```python
from build123d import *

# Parameters (mm, degrees)
F0_W      = 38.1
F0_H      = 6.35
F1_DEPTH  = 546.1
F3_DEPTH  = 12.7
F4_W      = 152.376732
F4_H      = 158.75
F5_DEPTH  = 50.8
F6_W      = 158.75
F6_H      = 12.7
F7_DEPTH  = 152.4
F8_W      = 6.35
F8_H      = 158.75
F9_DEPTH  = 12.7
F11_DEPTH = 152.4
F12_W     = 292.1
F12_H     = 44.45
F13_DEPTH = 139.7
F14_W     = 292.1
F14_H     = 44.45
F14_W_2   = 25.4
F14_H_2   = 12.7
F15_DEPTH = 6.35


with BuildPart() as f1:
    # F0 (on Top) → F1 (new body)
    with BuildSketch(Plane.XY):
        Polygon((-59.489019, 112.964728), (-59.489019, 100.264728), (-21.389019, 100.264728), (54.810981, 100.264728), (92.910981, 100.264728), (92.910981, 112.964728), align=None)
        with Locations((73.860981, 97.089728)):
            Rectangle(F0_W, F0_H)
        Polygon((92.910981, 93.914728), (54.810981, 93.914728), (42.110981, 93.914728), (42.110981, 68.514728), (92.910981, 68.514728), align=None)
        with Locations((-40.439019, 97.089728)):
            Rectangle(F0_W, F0_H)
        Polygon((-59.489019, 93.914728), (-59.489019, 68.514728), (-8.689019, 68.514728), (-8.689019, 93.914728), (-21.389019, 93.914728), align=None)
    extrude(amount=F1_DEPTH)

    # F2 (on face) → F3 (join)
    with BuildSketch(Plane(origin=(0, 0, 0), x_dir=(1, 0, 0), z_dir=(0, 0, -1))):
        Polygon((-59.489019, 45.785272), (-59.489019, -68.514728), (-8.689019, -68.514728), (42.110981, -68.514728), (92.910981, -68.514728), (92.910981, 45.785272), align=None)
    extrude(amount=-F3_DEPTH)

    # F4 (on face) → F5 (join)
    with BuildSketch(Plane(origin=(0, 0, 0), x_dir=(1, 0, 0), z_dir=(0, 0, -1))):
        with Locations((16.699347, -33.589728)):
            Rectangle(F4_W, F4_H)
    extrude(amount=F5_DEPTH)

    # F6 (on face) → F7 (join)
    with BuildSketch(Plane.YZ.offset(92.887713)):
        with Locations((33.589728, -44.45)):
            Rectangle(F6_W, F6_H)
    extrude(amount=F7_DEPTH)

    # F8 (on face) → F9 (join)
    with BuildSketch(Plane.XY.offset(-38.1)):
        with Locations((242.112713, 33.589728)):
            Rectangle(F8_W, F8_H)
    extrude(amount=F9_DEPTH)

    # F10 (on face) → F11 (join)
    with BuildSketch(Plane(origin=(-59.489019, 0, 0), x_dir=(0, -1, 0), z_dir=(-1, 0, 0))):
        Polygon((-112.964728, 12.7), (-112.964728, -50.8), (45.785272, -50.8), (45.785272, 12.7), (-68.514728, 12.7), align=None)
    extrude(amount=F11_DEPTH)

    # F12 (on face) → F13 (cut)
    with BuildSketch(Plane(origin=(0, 112.964728, 0), x_dir=(-1, 0, 0), z_dir=(0, 1, 0))):
        with Locations((59.489019, -15.875)):
            Rectangle(F12_W, F12_H)
    extrude(amount=-F13_DEPTH, mode=Mode.SUBTRACT)

    # F14 (on face) → F15 (join)
    with BuildSketch(Plane(origin=(0, 112.964728, 0), x_dir=(-1, 0, 0), z_dir=(0, 1, 0))):
        with Locations((59.489019, -15.875)):
            Rectangle(F14_W, F14_H)
        with Locations((59.489019, -15.875)):
            Rectangle(F14_W_2, F14_H_2, mode=Mode.SUBTRACT)
    extrude(amount=-F15_DEPTH)


solid = f1.part
```
The listing builds one solid part. Answer for the finished solid, in the listing's coordinates (mm). A direction names the side the tool comes from. Give positions to 0.01 mm unless a question says otherwise; leave off trailing zeros. Order: outer loops, then holes, each group sorted by start corner. A loop starts at its lowest first (then second) coordinate and runs counter-clockwise, first axis right, second up. Notation, with made-up numbers: (41.5, 46) - (60.5, 46) arc R24 cw to (60.5, 72) - close; hole circle Ø8 at (-28, 87.5). An arc over 180 degrees is marked (long way). Use one line per item in the form item = value. Start each with the question number.
(1) The mould has two halves that part along Z. Classify faces 5 (the flat face through (20, 35, -50.8)), 6 (the flat face through (-57, 41, -38.1)), 7 (the flat face through (42.111, 81, 272)): released by +Z, released by -Z, zero draft, split by the parting line, or undercut.
(2) A cutting plane is placed at D-D, the plane x = 22. Write down the section's boundary in (y, z).
(3) Flat-ended cylindrical pins translate along their axes: pin 1 Ø3 at (y, z) = (96.5, 371) entering from +X; pin 2 Ø3 at (x, y) = (240.5, 26.5) entering from +Z; pin 3 Ø1.9 at (y, z) = (97.5, 276) entering from -X. Find the tip coordinate at first contact, or state that the pin passes through.
(4) For faces 1 (the flat face through (92.888, 35, -19)), 2 (the flat face through (16, 100.265, 272)), 3 (the flat face through (92.911, 81, 252)), 4 (the flat face through (-57, 41, 6.35)), determine the directions among +Z, -Z, +X, -X, +Y, -Y from which every point of the face is accessible in a straight line to the end or side of a thin tool.
(5) A cutting plane is placed at A-A, the plane z = 100.5. Write down the section's boundary in (x, y), then the cut area to 3 significant figures.
(6) Consider line 1 (Z direction, x = -3, y = -10); line 2 (Y direction, x = 77, z = -12.5); line 3 (X direction, y = 77, z = 388). Determine where each line is inside the solid, lowest interval first. Write a range as from..to.
(7) A cutting plane is placed at C-C, the plane x = -91. Write down the section's boundary in (y, z).
Ans:
q1.face_5 = released by -Z
q1.face_6 = undercut
q1.face_7 = zero draft
q2.outline = (-45.79, -50.8) - (112.96, -50.8) - (112.96, 546.1) - (100.26, 546.1) - (100.26, 6.35) - (106.61, 6.35) - (106.61, -38.1) - (-26.74, -38.1) - (-26.74, 6.35) - (68.51, 6.35) - (68.51, 12.7) - (-45.79, 12.7) - close
q3.pin_1 = 92.91
q3.pin_2 = -25.4
q3.pin_3 = -59.49
q4.face_1 = +Z, +Y, -Y
q4.face_2 = +Z
q4.face_3 = +Z, +X, +Y, -Y
q4.face_4 = none
q5.outline = (-59.49, 68.51) - (-8.69, 68.51) - (-8.69, 93.91) - (-21.39, 93.91) - (-21.39, 100.26) - (54.81, 100.26) - (54.81, 93.91) - (42.11, 93.91) - (42.11, 68.51) - (92.91, 68.51) - (92.91, 112.96) - (-59.49, 112.96) - close
q5.area = 5,000 mm^2
q6.line_1 = -50.8..-38.1, 6.35..12.7
q6.line_2 = -45.79..-26.74, 106.61..112.96
q6.line_3 = -59.49..-8.69, 42.11..92.91
q7.outline = (-45.79, -50.8) - (112.96, -50.8) - (112.96, 12.7) - (-45.79, 12.7) - close; hole (-26.74, -38.1) - (106.61, -38.1) - (106.61, 6.35) - (-26.74, 6.35) - close
